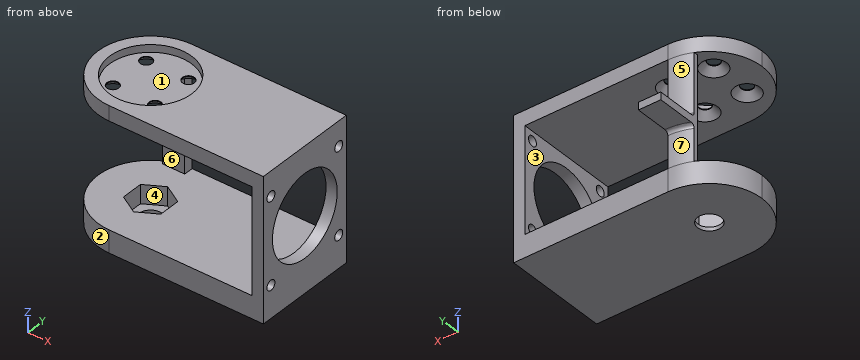
Autodesk Inventor part; units mm, degrees
ref_plane "工作平面4" through (3, -14.075, -3.53) normal (0, 0, 1) x (1, 0, 0)
ref_plane "YZ Plane" through (0, 0, 0) normal (1, 0, 0) x (0, 1, 0)
ref_plane "XZ Plane" through (0, 0, 0) normal (0, 1, 0) x (-1, 0, 0)
sketch "草圖1" plane through (0, 0, 0) normal (1, 0, 0) x (0, 1, 0)
  line L0 (-14.075, 14.075) -> (14.075, 14.075)
  line L1 (14.075, 14.075) -> (14.075, -14.075)
  line L2 (14.075, -14.075) -> (-14.075, -14.075)
  line L3 (-14.075, -14.075) -> (-14.075, 14.075)
  line L4 (-14.075, 14.075) -> (14.075, -14.075) construction
  line L5 (14.075, 14.075) -> (-14.075, -14.075) construction
  line L6 (14.075, 14.075) -> (-14.075, 14.075)
  line L7 (-14.075, 14.075) -> (-14.075, 18.075)
  line L8 (-14.075, 18.075) -> (14.075, 18.075)
  line L9 (14.075, 18.075) -> (14.075, 14.075)
  circle A0 centre (0, 0) radius 11
  line L10 (-11.5, 11.5) -> (11.5, 11.5) construction
  line L11 (11.5, 11.5) -> (11.5, -11.5) construction
  line L12 (11.5, -11.5) -> (-11.5, -11.5) construction
  line L13 (-11.5, -11.5) -> (-11.5, 11.5) construction
  line L14 (-11.5, 11.5) -> (11.5, -11.5) construction
  line L15 (11.5, 11.5) -> (-11.5, -11.5) construction
  circle A1 centre (11.5, 11.5) radius 1.35
  circle A2 centre (-11.5, 11.5) radius 1.35
  circle A3 centre (-11.5, -11.5) radius 1.35
  circle A4 centre (11.5, -11.5) radius 1.35
  line L16 (14.075, -14.075) -> (-14.075, -14.075)
  line L17 (-14.075, -14.075) -> (-14.075, -20.075)
  line L18 (-14.075, -20.075) -> (14.075, -20.075)
  line L19 (14.075, -20.075) -> (14.075, -14.075)
  dimension "d0" = 28.15
  dimension "d1" = 28.15
  dimension "d2" = 4
  dimension "d3" = 22
  dimension "d4" = 23
  dimension "d5" = 23
  dimension "d6" = 2.7
  dimension "d9" = 360
  dimension "d11" = 6
extrude "擠出1" add sketch "草圖1" along normal blind 3
sketch "草圖2" plane through (0, 0, 0) normal (-1, 0, 0) x (0, 0, 1)
  line L0 (18.075, 14.075) -> (18.075, -14.075)
  line L1 (-20.075, 14.075) -> (18.075, 14.075)
  line L2 (-20.075, -14.075) -> (-20.075, 14.075)
  line L3 (18.075, -14.075) -> (-20.075, -14.075)
  circle A0 centre (0, 0) radius 11
  circle A1 centre (11.5, 11.5) radius 1.35
  circle A2 centre (11.5, -11.5) radius 1.35
  circle A3 centre (-11.5, -11.5) radius 1.35
  circle A4 centre (-11.5, 11.5) radius 1.35
  line L4 (-14.075, 14.075) -> (-14.075, -14.075)
  line L5 (14.075, 14.075) -> (14.075, -14.075)
  dimension "d14" = 6
  dimension "d15" = 4
extrude "擠出2" add sketch "草圖2" along normal blind 52.375 contours L0 L3 L5 L1 | L4 L3 L2 L1
sketch "草圖3" plane through (3, -14.075, 18.075) normal (0, 0, 1) x (1, 0, 0)
  line L0 (-55.375, 0) -> (0, 0)
  line L1 (0, 28.15) -> (0, 0)
  line L2 (0, 28.15) -> (-55.375, 28.15)
  line L3 (-55.375, 0) -> (-55.375, 28.15)
  circle A0 centre (-41.3, 14.075) radius 11
  line L4 (-55.375, 0) -> (-55.375, 28.15)
  circle A1 centre (-41.3, 14.075) radius 8 construction
  line L5 (-41.3, 14.075) -> (-33.5218, 21.8532) construction
  line L6 (-41.3, 14.075) -> (-30.3, 14.075) construction
  circle A2 centre (-35.6431, 19.7319) radius 1.6
  circle A3 centre (-46.9569, 19.7319) radius 1.6
  circle A4 centre (-46.9569, 8.4181) radius 1.6
  circle A5 centre (-35.6431, 8.4181) radius 1.6
  point P0 (-3, 14.075)
  dimension "d18" = 22
  dimension "d19" = 16
  dimension "d65" = 10
  dimension "d20" = 45
  dimension "d21" = 3.2
  dimension "d24" = 360
  dimension "d30" = 14.075
  dimension "d31" = 14.075
extrude "擠出3" cut sketch "草圖3" against normal up to surface (4 mm away) contours A2 | A3 | A4 | A5
extrude "擠出4" cut sketch "草圖3" against normal blind 2 contours A0
fillet "圓角1" radius 14.075 4 edges at (-52.375, 14.075, 16.075) (-52.375, 14.075, -17.075) (-52.375, -14.075, 16.075) (-52.375, -14.075, -17.075)
sketch "草圖4" plane through (0, -14.075, -14.075) normal (0, 0, 1) x (1, 0, 0)
  circle A0 centre (-38.3, 14.075) radius 11
  line L0 (-38.3, 8.3015) -> (-43.3, 11.1882)
  line L1 (-43.3, 11.1882) -> (-43.3, 16.9618)
  line L2 (-43.3, 16.9618) -> (-38.3, 19.8485)
  line L3 (-38.3, 19.8485) -> (-33.3, 16.9618)
  line L4 (-33.3, 16.9618) -> (-33.3, 11.1882)
  line L5 (-33.3, 11.1882) -> (-38.3, 8.3015)
  point P0 (0, 14.075)
  dimension "d33" = 10
extrude "擠出5" cut sketch "草圖4" against normal blind 5 contours L0 L1 L2 L3 L4 L5
sketch "草圖5" plane through (0, -14.075, -19.075) normal (0, 0, 1) x (1, 0, 0)
  circle A0 centre (-38.3, 14.075) radius 11
  circle A1 centre (-38.3, 14.075) radius 3.1
  point P0 (0, 14.075)
  dimension "d36" = 6.2
extrude "擠出6" cut sketch "草圖5" against normal up to surface (1 mm away) contours A1
sketch "草圖7" plane through (3, 0, 0) normal (1, 0, 0) x (0, 0, -1)
  line L0 (-18.075, 14.075) -> (-18.075, -14.075)
  line L1 (-18.075, -14.075) -> (20.075, -14.075)
  line L2 (20.075, -14.075) -> (20.075, 14.075)
  line L3 (20.075, 14.075) -> (-18.075, 14.075)
  circle A0 centre (0, 0) radius 11
  circle A1 centre (-11.5, 11.5) radius 1.35
  circle A2 centre (-11.5, -11.5) radius 1.35
  circle A3 centre (11.5, -11.5) radius 1.35
  circle A4 centre (11.5, 11.5) radius 1.35
  line L4 (-2.75, 14.075) -> (-2.75, 10.6507)
  line L5 (2.75, 14.075) -> (2.75, 10.6507)
  dimension "d44" = 5.5
  dimension "d45" = 2.75
chamfer "倒角1" distance 1.8 angle 45 4 edges at (-45.5569, -5.6569, 14.075) (-45.5569, 5.6569, 14.075) (-34.2431, -5.6569, 14.075) (-34.2431, 5.6569, 14.075)
sketch "草圖11" plane through (3, -14.075, 18.075) normal (0, 0, 1) x (1, 0, 0)
  line L0 (-37.3248, 33.6873) -> (-37.3375, 43.4872)
  line L1 (-37.3248, 33.6873) -> (-31.2248, 33.6951)
  line L2 (-31.2375, 43.4951) -> (-31.2248, 33.6951)
  line L3 (-37.3375, 43.4872) -> (-31.2375, 43.4951)
  arc A0 (-41.3, 28.15) -> (-41.3, 0) centre (-41.3, 14.075) ccw
  line L4 (-41.3, 0) -> (0, 0)
  line L5 (0, 28.15) -> (0, 0)
  line L6 (0, 28.15) -> (-41.3, 28.15)
  circle A1 centre (-41.3, 14.075) radius 11
  line L7 (-31.2003, 28.15) -> (-31.2003, 25.65)
  line L8 (-31.2003, 25.65) -> (-47.301, 25.65)
  line L9 (-47.301, 25.65) -> (-47.301, 26.8066)
  line L10 (-41.3, 28.15) -> (-41.3, 25.65)
  point P0 (-3, 14.075)
  dimension "d64" = 2.5
extrude "擠出12" add sketch "草圖11" against normal up to surface (38.15 mm away) contours L10 L8 L9 A0
ref_plane "工作平面4" through (3, -14.075, -3.53) normal (0, 0, 1) x (1, 0, 0)
sketch "草圖15" plane through (3, -14.075, -3.53) normal (0, 0, 1) x (1, 0, 0)
  line L0 (0, 28.15) -> (-41.3, 28.15)
  arc A0 (-41.3, 28.15) -> (-41.3, 0) centre (-41.3, 14.075) ccw
  line L1 (-47.3274, 33.6866) -> (-47.3385, 41.6466) construction
  line L2 (-47.3274, 33.6866) -> (-41.2274, 33.6951) construction
  line L3 (-41.2385, 41.6551) -> (-41.2274, 33.6951) construction
  line L4 (-47.3385, 41.6466) -> (-41.2385, 41.6551) construction
  line L5 (-41.3, 38.15) -> (-47.301, 38.15)
  line L6 (-41.3, 38.15) -> (-41.3, 28.15)
  line L7 (-47.301, 38.15) -> (-47.301, 26.8066)
  point P0 (-3, 14.075)
  point P1 (-47.301, 26.8066)
  dimension "d78" = 10
extrude "擠出16" add sketch "草圖15" along normal mid plane 2
fillet "圓角5" radius 1 2 edges at (-41.3748, 13.735, -4.53) (-41.3748, 13.735, -2.53)
equation "\"d26\" = d19"
properties part number "j6 motor mount v2_3D 列印"
Input: part model. Units: mm. Frame: model coordinates. Face numbers are marked on the shaded views. A direction names the side the tool comes from. Give positions to 0.01 mm unless a question says otherwise; leave off trailing zeros. Loops run counter-clockwise (first coordinate to the right, second up) from the corner with the lowest first, then second, coordinate; pieces in that order, holes last. Notation, with made-up numbers: (6.25, 61.5) -> (45.25, 61.5) arc R22 ccw to (45.25, 85.5) -> close; hole circle Ø8 at (-24.5, 38.5). An arc over 180 degrees is marked (long way). Answer as a JSON object with one key per item and string values. Group by question number.
Item 1: Reachability of the marked faces 4, 5, 6 and 7 from +Z, -Z, +X, -X, +Y, -Y: full face, straight path, thin tool, end or side. Return the list, or none.
Item 2: Cut plane D-D, the plane y = 18.5. Return the cut outline in (x, z).
Item 3: Line query: probe 1 along Z at (x, y) = (-32, 11.5) (3 decimals); probe 2 along Y at (x, z) = (-38.3, 17.5) (3 decimals); probe 3 along Y at (x, z) = (-3, -15) (3 decimals). Output: solid intervals per line, ascending.
Item 4: Cut plane A-A, the plane x = -12. Return the cut outline in (y, z) (3 decimals).
Item 5: Cut plane C-C, the plane z = -7. Return the cut outline in (x, y) (3 decimals), and give its area (3 significant figures).
Item 6: Pull-direction query (Z, two-part tool) for the marked faces 1, 2 and 3; classes: released by +Z, released by -Z, zero draft, split by the parting line, or undercut.
Item 7: Pin query (flat end, axial travel): P1, Ø12, axis at y = 7, z = -11, coming from the -X side; P2, Ø5, axis at x = -40, z = 2, coming from the -Y side (3 decimals); P3, Ø12, axis at x = -24.5, z = -8.5, coming from the +Y side (3 decimals); P4, Ø2.5, axis at y = -11.5, z = -11.5, coming from the -X side. Return the tip coordinate at first contact, or that it passes through.
Checks:
{
 "1": {"face 4": "none", "face 5": "+Z, -X, +Y", "face 6": "-X, -Y", "face 7": "-Z, -X, +Y"},
 "2": {"outline": "(-44.3, -4.53) -> (-38.3, -4.53) -> (-38.3, -2.53) -> (-44.3, -2.53) -> close"},
 "3": {"probe 1": "z = -20.075 to -14.075, 14.075 to 18.075", "probe 2": "y = -14.075 to -11, 11 to 14.075", "probe 3": "y = -14.075 to 14.075"},
 "4": {"outline": "(-14.075, -20.075) -> (14.075, -20.075) -> (14.075, -14.075) -> (-14.075, -14.075) -> close; (-14.075, 14.075) -> (14.075, 14.075) -> (14.075, 18.075) -> (-14.075, 18.075) -> close"},
 "5": {"outline": "(-44.301, 11.575) -> (-38.3, 11.575) -> (-38.3, 14.075) arc R14.075 ccw to (-44.301, 12.732) -> close; (0, -14.075) -> (3, -14.075) -> (3, -8.485) -> (0, -8.485) -> close; (0, 8.485) -> (3, 8.485) -> (3, 14.075) -> (0, 14.075) -> close", "area": "45.9 mm²"},
 "6": {"face 1": "released by +Z", "face 2": "zero draft", "face 3": "undercut"},
 "7": {"P1": "stops at x = -52.25", "P2": "stops at y = 11.575", "P3": "stops at y = 14.075", "P4": "passes through"}
}
